from build123d import *

# Parameters (mm, degrees)
BOSS_EXTRUDE1_DEPTH = 1.5
SKETCH1_8_R         = 4.05
BOSS_EXTRUDE3_DEPTH = 36
SKETCH1_9_R         = 5.05
BOSS_EXTRUDE4_DEPTH = 19
SHELL1_START        = 2
SHELL1_OUTLINE_R    = 3.05
SHELL1_DEPTH        = 15
SHELL1_START_2      = 17
SHELL1_2_OUTLINE_R  = 2.05
SHELL1_2_DEPTH      = 17
SKETCH1_10_R        = 3.05
CUT_EXTRUDE1_DEPTH  = 11
SKETCH1_3_R         = 3.05
BOSS_EXTRUDE2_DEPTH = 6
CHAMFER1_SIZE       = 2
CHAMFER1_SIZE2      = 0.727940469
CHAMFER2_SIZE       = 2.747477419
CHAMFER2_SIZE_2     = 1
CHAMFER3_SIZE       = 1.039230485
CHAMFER3_SIZE_2     = 0.6
CHAMFER5_SIZE       = 0.3


# Read off the part's stored shape, not the designer's step: Shell1
with BuildPart() as part:
    # Sketch1 → Boss-Extrude1 (new body)
    with BuildSketch(Plane.XY):
        Polygon((-7.1, 4.099186911), (0, 8.198373822), (7.1, 4.099186911), (7.1, -4.099186911), (0, -8.198373822), (-7.1, -4.099186911), align=None)
    extrude(amount=BOSS_EXTRUDE1_DEPTH)

    # Sketch1<8> → Boss-Extrude3 (add)
    with BuildSketch(Plane.XY):
        with Locations(Location((0, 0, 0), (0, 0, 180))):
            Circle(SKETCH1_8_R)
    extrude(amount=BOSS_EXTRUDE3_DEPTH)

    # Sketch1<9> → Boss-Extrude4 (add)
    with BuildSketch(Plane.XY):
        with Locations(Location((0, 0, 0), (0, 0, 180))):
            Circle(SKETCH1_9_R)
    extrude(amount=BOSS_EXTRUDE4_DEPTH)

    # Shell1 outline → Shell1 (cut)
    with BuildSketch(Plane.XY.offset(SHELL1_START)):
        Circle(SHELL1_OUTLINE_R)
    extrude(amount=SHELL1_DEPTH, mode=Mode.SUBTRACT)

    # Shell1 2 outline → Shell1 2 (cut)
    with BuildSketch(Plane.XY.offset(SHELL1_START_2)):
        Circle(SHELL1_2_OUTLINE_R)
    extrude(amount=SHELL1_2_DEPTH, mode=Mode.SUBTRACT)

    # Sketch1<10> → Cut-Extrude1 (cut)
    with BuildSketch(Plane.XY):
        Circle(SKETCH1_10_R)
    extrude(amount=CUT_EXTRUDE1_DEPTH, mode=Mode.SUBTRACT)

    # Sketch1<3> → Boss-Extrude2 (add)
    with BuildSketch(Plane.XY):
        Polygon((0, 7.159143338), (6.2, 3.579571669), (6.2, -3.579571669), (0, -7.159143338), (-6.2, -3.579571669), (-6.2, 3.579571669), align=None)
        Circle(SKETCH1_3_R, mode=Mode.SUBTRACT)
    extrude(amount=BOSS_EXTRUDE2_DEPTH)

    # Chamfer1
    chamfer1_edges = [part.edges().sort_by_distance(p)[0] for p in [
        (4.05, 0, 36),
    ]]
    chamfer1_side = [part.faces().sort_by_distance(p)[0] for p in [
        (4.05, 0, 27.5),
    ]]
    chamfer(chamfer1_edges, length=CHAMFER1_SIZE, length2=CHAMFER1_SIZE2, reference=chamfer1_side[0])

    # Chamfer2
    # the kernel refuses this chamfer: 2.747477419, 1 mm, written as the material it adds along each edge
    with BuildSketch(Plane(origin=(0, 0, 19), x_dir=(-1, 0, 0), z_dir=(0, -1, 0))) as chamfer2_piece_1_section:
        Polygon((4.05, -CHAMFER2_SIZE), (4.05 + CHAMFER2_SIZE_2, 0), (4.05, 0), align=None)
    chamfer2_piece_1 = revolve(axis=Axis((0, 0, 19), (0, 0, -1)), mode=Mode.PRIVATE)
    chamfer2_piece_1 = chamfer2_piece_1 & Plane(origin=(0, 0, 20.413276919), x_dir=(-1, 0, 0), z_dir=(0, 0, -1)) * Cylinder(5.05, 21, mode=Mode.PRIVATE)
    add(chamfer2_piece_1)

    # Chamfer3
    # the kernel refuses this chamfer: 1.039230485, 0.6 mm, written as the material it takes off along each edge
    with BuildSketch(Plane(origin=(0, 0, 17), x_dir=(1, 0, 0), z_dir=(0, -1, 0))) as chamfer3_piece_1_section:
        Polygon((2.05 + CHAMFER3_SIZE, 0), (2.05, CHAMFER3_SIZE_2), (2.05, 0), align=None)
    chamfer3_piece_1 = revolve(axis=Axis((0, 0, 17), (0, 0, 1)), mode=Mode.PRIVATE)
    chamfer3_piece_1 = chamfer3_piece_1 & Plane(origin=(0, 0, 17.306641595), x_dir=(1, 0, 0), z_dir=(0, 0, -1)) * Cylinder(3.05, 13, mode=Mode.PRIVATE)
    add(chamfer3_piece_1, mode=Mode.SUBTRACT)

    # Chamfer5
    chamfer5_edges = [part.edges().sort_by_distance(p)[0] for p in [
        (3.55, 6.148780367, 1.5),
        (7.1, 0, 1.5),
        (3.55, -6.148780367, 1.5),
        (-3.55, -6.148780367, 1.5),
        (5.05, 0, 6),
        (-7.1, 0, 1.5),
        (-3.1, -5.369357503, 6),
        (3.1, -5.369357503, 6),
        (6.2, 0, 6),
        (3.1, 5.369357503, 6),
        (-3.1, 5.369357503, 6),
        (-6.2, 0, 6),
        (-3.55, 6.148780367, 1.5),
    ]]
    chamfer(chamfer5_edges, length=CHAMFER5_SIZE)


solid = part.part
Build history of the part. All positions in model axes, mm. A direction names the side the tool comes from. Give positions to 0.01 mm unless a question says otherwise; leave off trailing zeros. Order: outer loops, then holes, each group sorted by start corner. A loop starts at its lowest first (then second) coordinate and runs counter-clockwise, first axis right, second up. Notation, with made-up numbers: M -18.75,7.5 L 38.25,7.5 A20 ccw 38.25,32.5 Z; hole C 84.5,-31.5 d5. An arc over 180 degrees is marked long. Use one line per item in the form item = value.
1) Saw through at C-C (z = 32.5). Give the cut face in (x, y).
Calculated:
outline = C 0,0 d8.1; hole C 0,0 d4.1
2) Tool access for faces 5 (the face through (-6.2, 0, 4)), 6 (the face through (0.878, 3.954, 27.788)), 7 (the face through (3.057, 5.394, 3.571)), 8 (the face through (-3.057, -5.394, 3.571)), 9 (the face through (3.6, -6.12, 0.59)): list every direction of +Z, -Z, +X, -X, +Y, -Y with a clear straight run to the whole face (end or side of a thin tool).
Calculated:
face_5 = +Z, -X, +Y, -Y
face_6 = +Z
face_7 = +Z, +X, +Y
face_8 = +Z, -X, -Y
face_9 = +Z, -Z, +X, -Y
3) Saw through at D-D (z = 20.5). Give the cut face in (x, y).
Calculated:
outline = C 0,0 d9.01; hole C 0,0 d4.1
4) Two-plate mould, pull along Y, no slides. Class faces 1 (the face through (-0.267, 2.033, 25.685)), 2 (the face through (4, 4, 6)), 3 (the face through (0, 0, 34)), 4 (the face through (3.426, 6.049, 1.348)): released by +Y, released by -Y, zero draft, split by the parting line, or undercut.
Calculated:
face_1 = undercut
face_2 = zero draft
face_3 = undercut
face_4 = released by +Y
5) Probe probe 1 along Y at (x, z) = (0, 30.5); probe 2 along Y at (x, z) = (0, 7.5); probe 3 along X at (y, z) = (1.75, 23). List the from-to ranges inside material, lowest first.
Calculated:
probe_1 = -4.05 to -2.05, 2.05 to 4.05
probe_2 = -5.05 to -3.05, 3.05 to 5.05
probe_3 = -3.65 to -1.07, 1.07 to 3.65
6) Saw through at A-A (z = 4.5). Give the cut face in (x, y), plus the area to 3 significant figures.
Calculated:
outline = M -6.2,-3.58 L 0,-7.16 L 6.2,-3.58 L 6.2,3.58 L 0,7.16 L -6.2,3.58 Z; hole C 0,0 d6.1
area = 104 mm2
7) Drop flat-ended pins along their axis: pin 1 (4.5 mm diameter, centred on x = -1, y = 0.5, fed in from -Z); pin 2 (3.5 mm diameter, centred on x = 0, y = 0, fed in from -Z); pin 3 (1.3 mm diameter, centred on y = 0, z = 2.5, fed in from +X); pin 4 (3 mm diameter, centred on x = 3.5, z = 27.5, fed in from +Y). Give the stop position or say it passes through.
Calculated:
pin_1 = 0
pin_2 = 34
pin_3 = 6.2
pin_4 = 3.52
